Autodesk Inventor part; units mm, degrees
ref_plane "YZ Plane" through (0, 0, 0) normal (1, 0, 0) x (0, 1, 0)
ref_plane "XZ Plane" through (0, 0, 0) normal (0, 1, 0) x (-1, 0, 0)
ref_plane "XY Plane" through (0, 0, 0) normal (0, 0, 1) x (1, 0, 0)
sketch "Эскиз1" plane through (0, 0, 0) normal (0, 0, 1) x (1, 0, 0)
  line L0 (-178.396, -16.0989) -> (-159.396, -16.0989)
  arc A0 (-159.396, -16.0989) -> (-154.396, -11) centre (-159.395, -11.0989) ccw
  line L1 (-154.396, -11) -> (-154.396, 13.9011)
  arc A1 (-154.396, 13.9011) -> (-159.396, 18.9011) centre (-159.396, 13.9011) ccw
  line L2 (-159.396, 18.9011) -> (-178.396, 18.9011)
  circle A2 centre (-164.396, 11.4011) radius 1.5
  circle A3 centre (-164.396, -8.5989) radius 1.5
  line L3 (-178.396, -16.0989) -> (-178.396, 18.9011)
  point P0 (0, 0)
  dimension "d9" = 20
  dimension "d10" = 7.5
  dimension "d11" = 7.5
  dimension "d12" = 14
  dimension "d13" = 10
  dimension "d14" = 5
  dimension "d15" = 5
  dimension "d16" = 14
  dimension "d17" = 3
  dimension "d18" = 3
extrude "Выдавливание1" add sketch "Эскиз1" along normal blind 4
sketch "Эскиз2" plane through (0, 0, 4) normal (0, 0, 1) x (1, 0, 0)
  circle A0 centre (-164.396, -8.5989) radius 1.5
  circle A1 centre (-164.396, 11.4011) radius 1.5
  line L0 (-178.396, -16.0989) -> (-159.396, -16.0989)
  arc A2 (-159.396, -16.0989) -> (-154.396, -11) centre (-159.395, -11.0989) ccw
  line L1 (-154.396, -11) -> (-154.396, 13.9011)
  arc A3 (-154.396, 13.9011) -> (-159.396, 18.9011) centre (-159.396, 13.9011) ccw
  line L2 (-159.396, 18.9011) -> (-178.396, 18.9011)
  line L3 (-178.396, 18.9011) -> (-178.396, -16.0989)
  circle A4 centre (-164.396, -8.5989) radius 1.5
  line L4 (-167.6291, -8.5989) -> (-166.0125, -5.7989)
  line L5 (-166.0125, -5.7989) -> (-162.7794, -5.7989)
  line L6 (-162.7794, -5.7989) -> (-161.1628, -8.5989)
  line L7 (-161.1628, -8.5989) -> (-162.7794, -11.3989)
  line L8 (-162.7794, -11.3989) -> (-166.0125, -11.3989)
  line L9 (-166.0125, -11.3989) -> (-167.6291, -8.5989)
  line L10 (-167.6291, 11.4011) -> (-166.0125, 14.2011)
  line L11 (-166.0125, 14.2011) -> (-162.7794, 14.2011)
  line L12 (-162.7794, 14.2011) -> (-161.1628, 11.4011)
  line L13 (-161.1628, 11.4011) -> (-162.7794, 8.6011)
  line L14 (-162.7794, 8.6011) -> (-166.0125, 8.6011)
  line L15 (-166.0125, 8.6011) -> (-167.6291, 11.4011)
  line L16 (-159.396, 18.9011) -> (-178.396, 18.9011)
  line L17 (-178.396, -16.0989) -> (-159.396, -16.0989)
  point P0 (0, 0)
  point P1 (-164.396, 11.4011)
  dimension "d4" = 5.6
  dimension "d5" = 5.6
extrude "Выдавливание2" cut sketch "Эскиз2" against normal blind 2.5 contours L4 L5 L6 L7 L8 L9 | L10 L11 L12 L13 L14 L15
fillet "Сопряжение1" radius 2 8 edges at (-178.396, 1.4011, 4) (-155.825, -14.5996, 4) (-154.396, 1.4506, 4) (-155.8604, 17.4367, 4) (-168.896, 18.9011, 4) (-168.896, -16.0989, 4) (-178.396, -16.0989, 2) (-178.396, 18.9011, 2)
properties part number "крепление  магнитного замка"
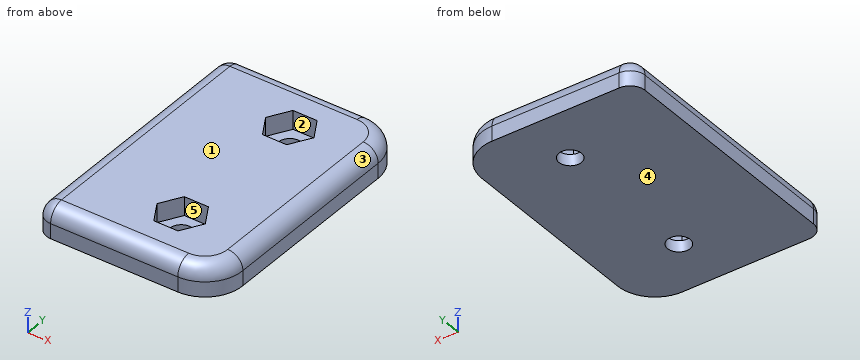
Could you check a few things on this model? Use its own coordinates, in mm. Face numbers are marked on the shaded views. A direction names the side the tool comes from. Round coordinates to 2 decimals unless told otherwise and drop trailing zeros. Loops run counter-clockwise (first coordinate to the right, second up) from the corner with the lowest first, then second, coordinate; pieces in that order, holes last. Notation, with made-up numbers: M 40.5,-39.5 L 88.5,-39.5 A18 cw 88.5,-17.5 Z; hole C 15,78.25 d5. An arc over 180 degrees is marked long. Write item = value, one per line.
1. I want a section at B-B, the plane y = 12. Write out the boundary of the cut face in (x, z).
Results below:
outline = M -178.4,0 L -165.77,0 L -165.77,1.5 L -167.28,1.5 L -167.28,4 L -176.4,4 A2 ccw -178.4,2 Z; M -163.02,0 L -154.4,0 L -154.4,2 A2 ccw -156.4,4 L -161.51,4 L -161.51,1.5 L -163.02,1.5 Z
2. I need wall thicknesses on probe 1 along Y at (x, z) = (-166, 2.1); probe 2 along Y at (x, z) = (-175.25, 2.1); probe 3 along Y at (x, z) = (-165.75, 3.15). Which ranges of each line are inside material? Lowest first, please.
Results below:
probe_1 = -16.1 to -11.4, -5.8 to 8.6, 14.2 to 18.9
probe_2 = -16.1 to 18.9
probe_3 = -15.74 to -11.4, -5.8 to 8.6, 14.2 to 18.54
3. Thinking about a two-plate mould opening in X: for the marked faces 1, 2 and 3, which applies, +X half, -X half, draft (parallel to the pull), parting line (faces both ways), or undercut?
Results below:
face_1 = draft
face_2 = undercut
face_3 = +X half
4. Which directions (+Z, -Z, +X, -X, +Y, -Y) give clear straight access to the entire face, cutting with the end or side of a thin tool? Please do the marked faces 4 and 5.
Results below:
face_4 = -Z, +X, -X, +Y, -Y
face_5 = +Z
5. I want a section at A-A, the plane x = -165.5. Write out the boundary of the cut face in (y, z).
Results below:
outline = M -16.1,0 L -9.61,0 L -9.61,1.5 L -11.4,1.5 L -11.4,4 L -14.1,4 A2 ccw -16.1,2 Z; M -7.58,0 L 10.39,0 L 10.39,1.5 L 8.6,1.5 L 8.6,4 L -5.8,4 L -5.8,1.5 L -7.58,1.5 Z; M 12.42,0 L 18.9,0 L 18.9,2 A2 ccw 16.9,4 L 14.2,4 L 14.2,1.5 L 12.42,1.5 Z
6. I want a section at D-D, the plane y = 7.5. Write out the boundary of the cut face in (x, z), and give its area (3 significant figures).
Results below:
outline = M -178.4,0 L -154.4,0 L -154.4,2 A2 ccw -156.4,4 L -176.4,4 A2 ccw -178.4,2 Z
area = 94.3 mm²
7. I want a section at C-C, the plane z = 3.05. Write out the boundary of the cut face in (x, y), and give its area (3 significant figures).
Results below:
outline = M -178.1,-14.1 A1.7 ccw -176.4,-15.8 L -159.4,-15.8 A4.7 ccw -154.69,-11.01 L -154.69,13.9 A4.7 ccw -159.4,18.6 L -176.4,18.6 A1.7 ccw -178.1,16.9 Z; hole M -167.63,-8.6 L -166.01,-11.4 L -162.78,-11.4 L -161.16,-8.6 L -162.78,-5.8 L -166.01,-5.8 Z; hole M -167.63,11.4 L -166.01,8.6 L -162.78,8.6 L -161.16,11.4 L -162.78,14.2 L -166.01,14.2 Z
area = 740 mm²
8. Will these pins go through, and if not, where does the flat tip stop? P1, Ø3, axis at x = -164.5, y = -8, coming from the +Z side; P2, Ø1.5, axis at x = -170.5, z = 2.5, coming from the -Y side; P3, Ø2.5, axis at x = -164.4, y = -8.6, coming from the +Z side; P4, Ø0.8, axis at x = -164, z = 2.5, coming from the +Y side.
Results below:
P1 = 1.5
P2 = -16.1
P3 = through
P4 = 18.9
